The drawing under review shows one solid part. Ordinate dimensions are in mm from its lowest x, y, z. Round coordinates to 2 decimals unless told otherwise and drop trailing zeros. Order: outer loops, then holes, each group sorted by start corner. A loop starts at its lowest first (then second) coordinate and runs counter-clockwise, first axis right, second up. Notation, with made-up numbers: M 77,74.25 L 96,74.25 A27 cw 96,113.25 Z; hole C -16,-28 d11. An arc over 180 degrees is marked long. Answer in a Markdown table with one row per item. Add a question column.
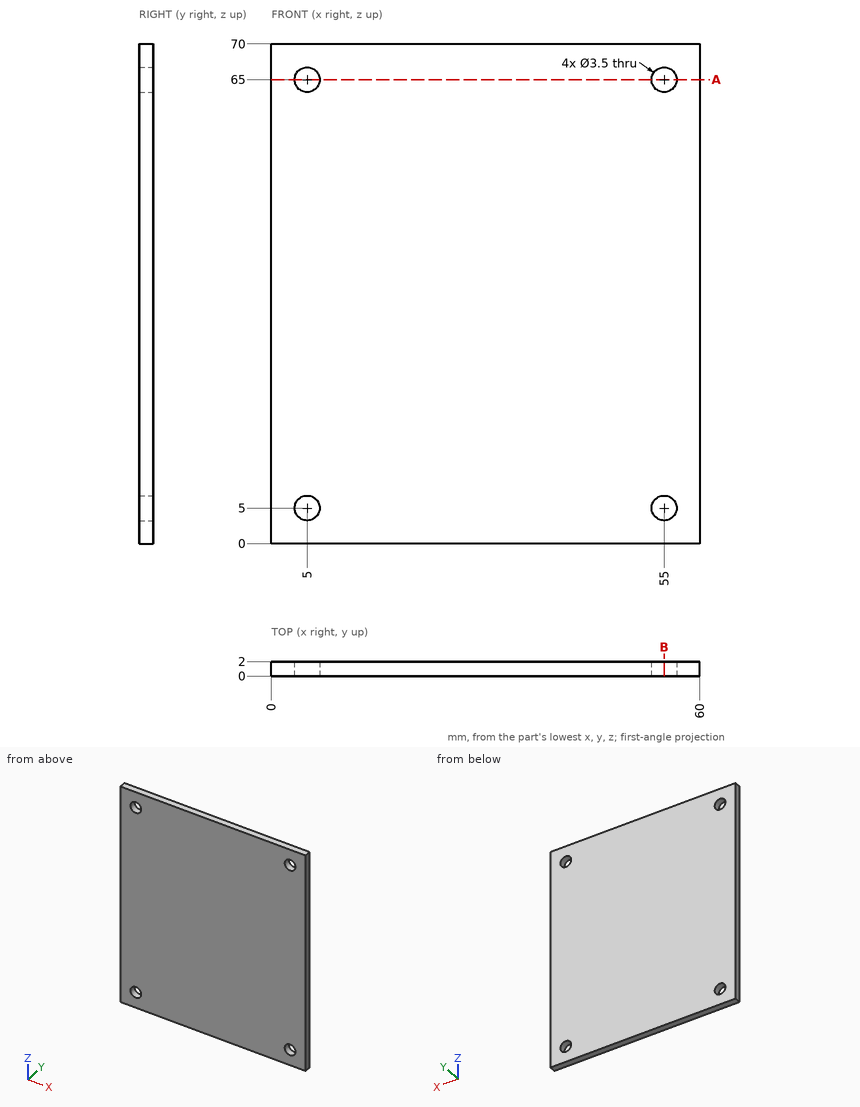
1. Consider section A-A on z = 65. Write out the cut boundary in (x, y), plus the area to 3 significant figures.
2. To check wall thickness, follow probe 1 along Z at (x, y) = (55, 0.7); probe 2 along X at (y, z) = (1.5, 65); probe 3 along Z at (x, y) = (53.5, 1.1). State the ranges of each line that lie inside material, in increasing order. Write a range as [from, to].
3. Clearance check with a flat-ended pin moving along its axis: pin 1 Ø3 at (x, z) = (55, 5) entering from -Y. State where the tip first meets the part, or that it passes through.
4. Consider section B-B on x = 55. Write out the cut boundary in (y, z), plus the area to 3 significant figures.
Solved:
| question | item | result |
|---|---|---|
| 1 | outline | M 0,0 L 3.25,0 L 3.25,2 L 0,2 Z; M 6.75,0 L 53.25,0 L 53.25,2 L 6.75,2 Z; M 56.75,0 L 60,0 L 60,2 L 56.75,2 Z |
| 1 | area | 106 mm^2 |
| 2 | probe 1 | z = [0, 3.25], [6.75, 63.25], [66.75, 70] |
| 2 | probe 2 | x = [0, 3.25], [6.75, 53.25], [56.75, 60] |
| 2 | probe 3 | z = [0, 4.1], [5.9, 64.1], [65.9, 70] |
| 3 | pin 1 | passes through |
| 4 | outline | M 0,0 L 2,0 L 2,3.25 L 0,3.25 Z; M 0,6.75 L 2,6.75 L 2,63.25 L 0,63.25 Z; M 0,66.75 L 2,66.75 L 2,70 L 0,70 Z |
| 4 | area | 126 mm^2 |
